from build123d import *

# Parameters (mm, degrees)
ESBO_O1_W                = 65
ESBO_O1_H                = 42
RESSALTO_EXTRUS_O1_DEPTH = 55
ESBO_O2_W                = 42
ESBO_O2_H                = 50
CORTE_EXTRUS_O1_DEPTH    = 10
ESBO_O3_W                = 42
ESBO_O3_H                = 42
CORTE_EXTRUS_O2_DEPTH    = 50
ESBO_O4_R                = 1.75
CORTE_EXTRUS_O3_DEPTH    = 78.239886069
ESBO_O5_R                = 1.75
CORTE_EXTRUS_O4_DEPTH    = 64.223808806
ESBO_O6_R                = 1.75
CORTE_EXTRUS_O5_DEPTH    = 58.107355043
ESBO_O7_R                = 3
CORTE_EXTRUS_O6_DEPTH    = 8
ESBO_O8_R                = 15
CORTE_EXTRUS_O7_DEPTH    = 78.239886069


with BuildPart() as part:
    # Esboço1 → Ressalto-extrusão1 (new body)
    with BuildSketch(Plane(origin=(0, 0, 0), x_dir=(1, 0, 0), z_dir=(0, 1, 0))):
        Rectangle(ESBO_O1_W, ESBO_O1_H)
    extrude(amount=RESSALTO_EXTRUS_O1_DEPTH)

    # Esboço2 → Corte-extrusão1 (cut)
    with BuildSketch(Plane.ZY.offset(32.5)):
        with Locations((0, 30)):
            Rectangle(ESBO_O2_W, ESBO_O2_H)
    extrude(amount=-CORTE_EXTRUS_O1_DEPTH, mode=Mode.SUBTRACT)

    # Esboço3 → Corte-extrusão2 (cut)
    with BuildSketch(Plane(origin=(32.5, 0, 0), x_dir=(0, 0, -1), z_dir=(1, 0, 0))):
        with Locations((0, 34)):
            Rectangle(ESBO_O3_W, ESBO_O3_H)
    extrude(amount=-CORTE_EXTRUS_O2_DEPTH, mode=Mode.SUBTRACT)

    # Esboço4 → Corte-extrusão3 (cut, through all)
    with BuildSketch(Plane(origin=(-17.5, 0, 0), x_dir=(0, 0, -1), z_dir=(1, 0, 0))):
        with Locations((-15.5, 49.5)):
            Circle(ESBO_O4_R)
        with Locations((15.5, 49.5)):
            Circle(ESBO_O4_R)
        with Locations((15.5, 19.070664067)):
            Circle(ESBO_O4_R)
        with Locations((-15.5, 18.5)):
            Circle(ESBO_O4_R)
    extrude(amount=-CORTE_EXTRUS_O3_DEPTH, mode=Mode.SUBTRACT)

    # Esboço5 → Corte-extrusão4 (cut, through all)
    with BuildSketch(Plane(origin=(0, 5, 0), x_dir=(1, 0, 0), z_dir=(0, 1, 0))):
        with Locations(Location((-27.5, 15.5, 0), (0, 0, 270))):
            Circle(ESBO_O5_R)
        with Locations(Location((-27.5, -15.5, 0), (0, 0, 270))):
            Circle(ESBO_O5_R)
    extrude(amount=-CORTE_EXTRUS_O4_DEPTH, mode=Mode.SUBTRACT)

    # Esboço6 → Corte-extrusão5 (cut, through all)
    with BuildSketch(Plane(origin=(0, 13, 0), x_dir=(1, 0, 0), z_dir=(0, 1, 0))):
        with Locations(Location((-12.5, 15.5, 0), (0, 0, 270))):
            Circle(ESBO_O6_R)
        with Locations(Location((27.5, 15.5, 0), (0, 0, 270))):
            Circle(ESBO_O6_R)
        with Locations(Location((27.5, -15.5, 0), (0, 0, 270))):
            Circle(ESBO_O6_R)
        with Locations(Location((-12.5, -15.5, 0), (0, 0, 270))):
            Circle(ESBO_O6_R)
    extrude(amount=-CORTE_EXTRUS_O5_DEPTH, mode=Mode.SUBTRACT)

    # Esboço7 → Corte-extrusão6 (cut)
    with BuildSketch(Plane(origin=(0, 13, 0), x_dir=(1, 0, 0), z_dir=(0, 1, 0))):
        with Locations(Location((-12.5, 15.5, 0), (0, 0, 270))):
            Circle(ESBO_O7_R)
        with Locations(Location((27.5, 15.5, 0), (0, 0, 270))):
            Circle(ESBO_O7_R)
        with Locations(Location((27.5, -15.5, 0), (0, 0, 270))):
            Circle(ESBO_O7_R)
        with Locations(Location((-12.5, -15.5, 0), (0, 0, 270))):
            Circle(ESBO_O7_R)
    extrude(amount=-CORTE_EXTRUS_O6_DEPTH, mode=Mode.SUBTRACT)

    # Esboço8 → Corte-extrusão7 (cut, through all)
    with BuildSketch(Plane(origin=(-17.5, 0, 0), x_dir=(0, 0, -1), z_dir=(1, 0, 0))):
        with Locations((0, 34)):
            Circle(ESBO_O8_R)
    extrude(amount=-CORTE_EXTRUS_O7_DEPTH, mode=Mode.SUBTRACT)


solid = part.part
Verification items for the finished model (mm, model axes). A direction names the side the tool comes from. Round coordinates to 2 decimals unless told otherwise and drop trailing zeros. Loops run counter-clockwise (first coordinate to the right, second up) from the corner with the lowest first, then second, coordinate; pieces in that order, holes last. Notation, with made-up numbers: (45, 19.5) - (55, 19.5) arc R17 cw to (55, 33.5) - close; hole circle Ø3 at (77.25, 87.5). An arc over 180 degrees is marked (long way). Use a Markdown table: item, result. Add a question column.
1. Thickness scan on probe 1 along Y at (x, z) = (-19.9, 15.5); probe 2 along X at (y, z) = (20.5, 12.5); probe 3 along Y at (x, z) = (11.5, 16). Record the ranges inside material, lowest first. Write a range as [from, to].
2. Release check for a two-part mould opening along Z. For faces 4 (the face through (-5, 11, -21)), 5 (the face through (27.6, 9.1, -18.5)), 6 (the face through (-20, 55, 0)) record: released by +Z, released by -Z, zero draft, split by the parting line, or undercut.
3. Access from +Z, -Z, +X, -X, +Y, -Y to the whole of each face (thin tool, end or side, straight path). Record for faces 1 (the face through (-28, 5, 0)), 2 (the face through (-12.4, 9.1, 12.5)), 3 (the face through (8, 13, 0)).
4. Gauge pin test, flat ends, axial feed: pin 1 (4 mm diameter, centred on y = 49.5, z = -15.5, fed in from +X); pin 2 (6.5 mm diameter, centred on x = 26.5, z = -14.5, fed in from +Y); pin 3 (4 mm diameter, centred on y = 31, z = -14.5, fed in from -X). Record the tip position at first contact, or that the pin passes through.
5. Section check B-B, the plane x = -27.5. Record the boundary of the cut face in (y, z).
6. Section check D-D, the plane y = 7. Record the boundary of the cut face in (x, z).
7. Section check C-C, the plane y = 34. Record the boundary of the cut face in (x, z), plus the area to 3 significant figures.
8. Section check A-A, the plane z = 0. Record the boundary of the cut face in (x, y).
Checks:
| question | item | result |
|---|---|---|
| 1 | probe 1 | y = [0, 16.75], [20.25, 47.75], [51.25, 55] |
| 1 | probe 2 | x = [-22.5, -17.5] |
| 1 | probe 3 | y = [0, 13] |
| 2 | face 4 | released by -Z |
| 2 | face 5 | undercut |
| 2 | face 6 | zero draft |
| 3 | face 1 | +Z, -Z, -X, +Y |
| 3 | face 2 | +Y |
| 3 | face 3 | +Z, -Z, +X, +Y |
| 4 | pin 1 | stops at x = -17.5 |
| 4 | pin 2 | stops at y = 13 |
| 4 | pin 3 | stops at x = -22.5 |
| 5 | outline | (0, -21) - (5, -21) - (5, -17.25) - (0, -17.25) - close; (0, -13.75) - (5, -13.75) - (5, 13.75) - (0, 13.75) - close; (0, 17.25) - (5, 17.25) - (5, 21) - (0, 21) - close |
| 6 | outline | (-22.5, -21) - (32.5, -21) - (32.5, 21) - (-22.5, 21) - close; hole circle Ø6 at (-12.5, -15.5); hole circle Ø6 at (-12.5, 15.5); hole circle Ø6 at (27.5, -15.5); hole circle Ø6 at (27.5, 15.5) |
| 7 | outline | (-22.5, -21) - (-17.5, -21) - (-17.5, -15) - (-22.5, -15) - close; (-22.5, 15) - (-17.5, 15) - (-17.5, 21) - (-22.5, 21) - close |
| 7 | area | 60.0 mm^2 |
| 8 | outline | (-32.5, 0) - (32.5, 0) - (32.5, 13) - (-17.5, 13) - (-17.5, 19) - (-22.5, 19) - (-22.5, 5) - (-32.5, 5) - close; (-22.5, 49) - (-17.5, 49) - (-17.5, 55) - (-22.5, 55) - close |
